Check sheet for the modelled part. Datum: model origin and axes. Units: mm. Face numbers are marked on the shaded views. A direction names the side the tool comes from. Coordinates: 2 decimals unless noted, no trailing zeros. Loops run counter-clockwise (first coordinate to the right, second up) from the corner with the lowest first, then second, coordinate; pieces in that order, holes last. Notation, with made-up numbers: (58.5, 67.5) - (96.5, 67.5) arc R18 ccw to (96.5, 100.5) - close; hole circle Ø2 at (29, 40.5). An arc over 180 degrees is marked (long way). Answer as a JSON object with one key per item and string values. Group by question number.
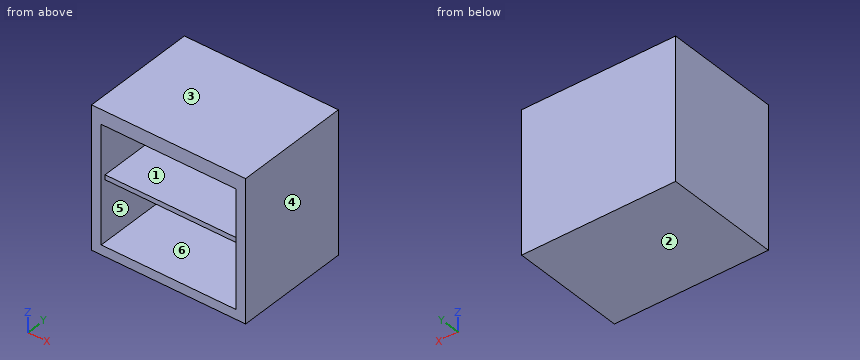
from build123d import *

# Parameters (mm, degrees)
F0_W     = 457.2
F0_H     = 558.8
F1_DEPTH = 609.6
F2_W     = 533.4
F2_H     = 463.55
F3_DEPTH = 444.5
F4_W     = 533.4
F4_H     = 19.05
F5_DEPTH = 425.45


# Not quite as in the source:
# - a feature names something its author has since deleted; it is built from what else it names


with BuildPart() as f1:
    # F0 (on Right) → F1 (new body)
    with BuildSketch(Plane.YZ):
        with Locations((-228.6, 279.4)):
            Rectangle(F0_W, F0_H)
    extrude(amount=F1_DEPTH)

    # F2 (on face) → F3 (cut)
    with BuildSketch(Plane.XZ.offset(457.2)):
        with Locations((304.8, 269.875)):
            Rectangle(F2_W, F2_H)
    extrude(amount=-F3_DEPTH, mode=Mode.SUBTRACT)

    # F4 (on face) → F5 (join)
    with BuildSketch(Plane.XZ.offset(12.7)):
        with Locations((304.8, 287.1150959969)):
            Rectangle(F4_W, F4_H)
    extrude(amount=F5_DEPTH)


solid = f1.part
1. Release check for a two-part mould opening along X. For the marked faces 3, 4, 5 and 6 record: released by +X, released by -X, zero draft, split by the parting line, or undercut.
2. Access from +Z, -Z, +X, -X, +Y, -Y to the whole of each face (thin tool, end or side, straight path). Record for the marked faces 1 and 2.
3. Sectioned sample at C-C on z = 450. Record the cut outline in (x, y), plus the area to 3 significant figures.
4. Sectioned sample at B-B on x = 346.5. Record the cut outline in (y, z), plus the area to 3 significant figures.
5. Sectioned sample at A-A on y = -276.5. Record the cut outline in (x, z), plus the area to 3 significant figures.
6. Gauge pin test, flat ends, axial feed: pin 1 (5 mm diameter, centred on x = 288, z = 374, fed in from -Y); pin 2 (15 mm diameter, centred on x = 356, z = 282.5, fed in from -Y). Record the tip position at first contact, or that the pin passes through.
7. Material ranges on line 1 (Z direction, x = 98, y = -42.5); line 2 (X direction, y = -206, z = 301); line 3 (Y direction, x = 149, z = 222), recorded low to high.
Answers follow:
{
 "1": {"face 3": "zero draft", "face 4": "released by +X", "face 5": "undercut", "face 6": "undercut"},
 "2": {"face 1": "-Y", "face 2": "-Z, +X, -X, +Y, -Y"},
 "3": {"outline": "(0, -457.2) - (38.1, -457.2) - (38.1, -12.7) - (571.5, -12.7) - (571.5, -457.2) - (609.6, -457.2) - (609.6, 0) - (0, 0) - close", "area": "41,600 mm^2"},
 "4": {"outline": "(-457.2, 0) - (0, 0) - (0, 558.8) - (-457.2, 558.8) - (-457.2, 501.65) - (-12.7, 501.65) - (-12.7, 296.64) - (-438.15, 296.64) - (-438.15, 277.59) - (-12.7, 277.59) - (-12.7, 38.1) - (-457.2, 38.1) - close", "area": "57,500 mm^2"},
 "5": {"outline": "(0, 0) - (609.6, 0) - (609.6, 558.8) - (0, 558.8) - close; hole (38.1, 38.1) - (571.5, 38.1) - (571.5, 277.59) - (38.1, 277.59) - close; hole (38.1, 296.64) - (571.5, 296.64) - (571.5, 501.65) - (38.1, 501.65) - close", "area": "104,000 mm^2"},
 "6": {"pin 1": "stops at y = -12.7", "pin 2": "stops at y = -438.15"},
 "7": {"line 1": "z = 0 to 38.1, 277.59 to 296.64, 501.65 to 558.8", "line 2": "x = 0 to 38.1, 571.5 to 609.6", "line 3": "y = -12.7 to 0"}
}
